CAD build for the part. Positions are in the model's coordinates, mm. Face numbers are marked on the shaded views. A direction names the side the tool comes from. Give positions to 0.01 mm unless a question says otherwise; leave off trailing zeros. Loops run counter-clockwise (first coordinate to the right, second up) from the corner with the lowest first, then second, coordinate; pieces in that order, holes last. Notation, with made-up numbers: M -3,31.25 L 32,31.25 A23 cw 32,65.25 Z; hole C 88.25,2.25 d5. An arc over 180 degrees is marked long. One line per question, with ' | ' between items.
```python
from build123d import *

# Parameters (mm, degrees)
EXTRUDE_1_DEPTH     = 15
CUT_EXTRUDE_1_REACH = 150.408
SKETCH_2_R          = 1.5
FILLET_2_R          = 3
SKETCH_3_R          = 3
CUT_EXTRUDE_2_DEPTH = 151.884061451


with BuildPart() as part:
    # 草图1 → 凸台-拉伸1 (new, symmetric)
    with BuildSketch(Plane.XY):
        Polygon((0, 0), (146, 0), (146, 28.5), (140.5, 28.5), (140.5, 13), (5.5, 13), (5.5, 35), (0, 35), align=None)
    extrude(amount=EXTRUDE_1_DEPTH, both=True)

    # 草图2 → 切除-拉伸1 (cut, up to next)
    with BuildSketch(Plane(origin=(0, 13, 0), x_dir=(1, 0, 0), z_dir=(0, 1, 0)), mode=Mode.PRIVATE) as cut_extrude_1_sk1:
        with Locations(Location((25.5, 8.5, 0), (0, 0, 180))):
            Circle(SKETCH_2_R)
    cut_extrude_1_tool1 = extrude(cut_extrude_1_sk1.sketch, amount=-CUT_EXTRUDE_1_REACH, mode=Mode.PRIVATE) & part.part
    # 草图2 → 切除-拉伸1 (cut, up to next)
    with BuildSketch(Plane(origin=(0, 13, 0), x_dir=(1, 0, 0), z_dir=(0, 1, 0)), mode=Mode.PRIVATE) as cut_extrude_1_sk2:
        with Locations(Location((120.5, 8.5, 0), (0, 0, 270))):
            Circle(SKETCH_2_R)
    cut_extrude_1_tool2 = extrude(cut_extrude_1_sk2.sketch, amount=-CUT_EXTRUDE_1_REACH, mode=Mode.PRIVATE) & part.part
    # 草图2 → 切除-拉伸1 (cut, up to next)
    with BuildSketch(Plane(origin=(0, 13, 0), x_dir=(1, 0, 0), z_dir=(0, 1, 0)), mode=Mode.PRIVATE) as cut_extrude_1_sk3:
        with Locations(Location((25.5, -8.5, 0), (0, 0, 270))):
            Circle(SKETCH_2_R)
    cut_extrude_1_tool3 = extrude(cut_extrude_1_sk3.sketch, amount=-CUT_EXTRUDE_1_REACH, mode=Mode.PRIVATE) & part.part
    # 草图2 → 切除-拉伸1 (cut, up to next)
    with BuildSketch(Plane(origin=(0, 13, 0), x_dir=(1, 0, 0), z_dir=(0, 1, 0)), mode=Mode.PRIVATE) as cut_extrude_1_sk4:
        with Locations(Location((120.5, -8.5, 0), (0, 0, 180))):
            Circle(SKETCH_2_R)
    cut_extrude_1_tool4 = extrude(cut_extrude_1_sk4.sketch, amount=-CUT_EXTRUDE_1_REACH, mode=Mode.PRIVATE) & part.part
    add(cut_extrude_1_tool1.solids().sort_by_distance((25.5, 13, -8.5))[0], mode=Mode.SUBTRACT)
    add(cut_extrude_1_tool2.solids().sort_by_distance((120.5, 13, -8.5))[0], mode=Mode.SUBTRACT)
    add(cut_extrude_1_tool3.solids().sort_by_distance((25.5, 13, 8.5))[0], mode=Mode.SUBTRACT)
    add(cut_extrude_1_tool4.solids().sort_by_distance((120.5, 13, 8.5))[0], mode=Mode.SUBTRACT)

    # 圆角2
    fillet_2_edges = [part.edges().sort_by_distance(p)[0] for p in [
        (143.25, 28.5, -15),
        (143.25, 28.5, 15),
        (2.75, 35, 15),
        (2.75, 35, -15),
    ]]
    fillet(fillet_2_edges, radius=FILLET_2_R)

    # 草图3 → 切除-拉伸2 (cut, through all)
    with BuildSketch(Plane.ZY):
        with Locations(Location((0, 20, 0), (0, 0, 270))):
            Circle(SKETCH_3_R)
    extrude(amount=-CUT_EXTRUDE_2_DEPTH, mode=Mode.SUBTRACT)


solid = part.part
```
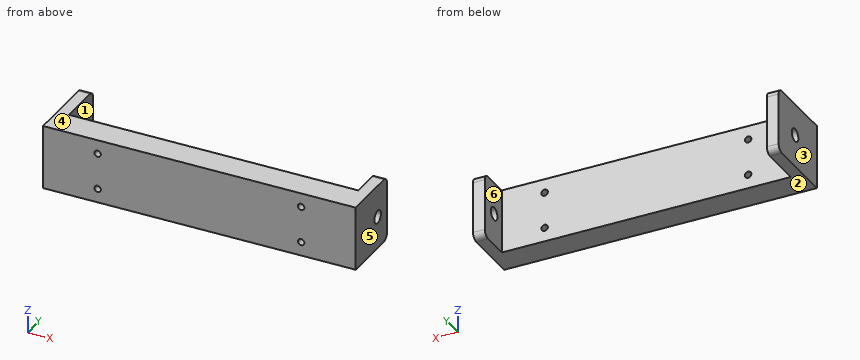
Item 1: 3-axis set-ups, long thin cutter, end or side, ignore diameter. For the marked faces 1 and 2: which of +Z, -Z, +X, -X, +Y, -Y reach the whole face in a straight line?
Conclusion:
face 1: +Z, -Z, +Y | face 2: -Z, +X, -X, +Y, -Y
Item 2: Drill centre lines: line 1 along Z through (x, y) = (120.5, 8); line 2 along X through (y, z) = (14, 5.5); line 3 along Z through (x, y) = (25, 4). Where is each one in solid material? Low to high. Write a range as [from, to].
Conclusion:
line 1: [-15, -10], [-7, 7], [10, 15] | line 2: [0, 5.5], [140.5, 146] | line 3: [-15, -9.91], [-7.09, 7.09], [9.91, 15]
Item 3: Saw through at A-A on z = 0. Give the cut face in (x, y).
Conclusion:
outline: M 0,0 L 146,0 L 146,17 L 140.5,17 L 140.5,13 L 5.5,13 L 5.5,17 L 0,17 Z; M 0,23 L 5.5,23 L 5.5,35 L 0,35 Z; M 140.5,23 L 146,23 L 146,28.5 L 140.5,28.5 Z
Item 4: Drop flat-ended pins along their axis: P1, Ø2, axis at y = 13, z = -11.5, coming from the -X side; P2, Ø4.5, axis at x = 144.5, z = 2, coming from the +Y side; P3, Ø1.5, axis at x = 24.5, z = -10.5, coming from the +Y side. Give the stop position or say it passes through.
Conclusion:
P1: x = 0 | P2: y = 28.5 | P3: y = 13
Item 5: Saw through at B-B on x = 120.5. Give the cut face in (y, z).
Conclusion:
outline: M 0,-15 L 13,-15 L 13,-10 L 0,-10 Z; M 0,-7 L 13,-7 L 13,7 L 0,7 Z; M 0,10 L 13,10 L 13,15 L 0,15 Z
Item 6: Mould opens along X. For the marked faces 3, 4, 5 and 6 say: pulls with the +X half, pulls with the -X half, needs draft (parallel to the pull), parting line crosses it, or undercut.
Conclusion:
face 3: pulls with the -X half | face 4: needs draft | face 5: pulls with the +X half | face 6: undercut
Item 7: Saw through at C-C on z = -8.5. Give the cut face in (x, y), and give its area (3 significant figures).
Conclusion:
outline: M 0,0 L 24,0 L 24,13 L 5.5,13 L 5.5,35 L 0,35 Z; M 27,0 L 119,0 L 119,13 L 27,13 Z; M 122,0 L 146,0 L 146,28.5 L 140.5,28.5 L 140.5,13 L 122,13 Z | area: 2,030 mm²
